Read the model definition and answer for the solid it produces. Units are mm, in the model's axes. A direction names the side the tool comes from. Round coordinates to 2 decimals unless told otherwise and drop trailing zeros. Write each loop counter-clockwise with the first axis right and the second up, starting at its lowest first coordinate (ties: lowest second). Pieces come first, ordered by that corner, then holes. Notation, with made-up numbers: (-17.75, 6.25) - (38.25, 6.25) arc R18 cw to (38.25, 28.25) - close; hole circle Ø1 at (-20.75, -27.75). An arc over 180 degrees is marked (long way). One line per item, written item: value. Start each with the question number.
(1) The mould has two halves that part along Y. Classify faces 1 (the face through (-35.587, -15.804, 3.451)), 2 (the face through (37.801, -21.974, 3.451)), 3 (the face through (1.2, -13.95, 3.45)): +Y half, -Y half, draft (parallel to the pull), parting line (faces both ways), or undercut.
(2) A cutting plane is placed at C-C, the plane x = -30. Determine the outline of the cut face in (y, z), plus the area to 3 significant figures.
(3) Flat-ended cylindrical pins translate along their axes: pin 1 Ø1.5 at (y, z) = (4.5, 5.5) entering from +X; pin 2 Ø1.5 at (y, z) = (1.5, 2) entering from +X; pin 3 Ø3 at (y, z) = (36, 6) entering from -X. Find the tip coordinate at first contact, or state that the pin passes through.
(4) Find the intervals of material crossed by L1, parallel to X at y = 1.5, z = 1.5; L2, parallel to X at y = 24, z = 5.5; L3, parallel to X at y = -15, z = 1, in increasing order.
(5) For faces 4 (the face through (8.566, -17.341, 3.451)), 5 (the face through (-16.806, -14.44, 3.451)), 6 (the face through (12.26, 6.76, 3.45)), determine the directions among +Z, -Z, +X, -X, +Y, -Y from which every point of the face is accessible in a straight line to the end or side of a thin tool.
(6) A cutting plane is placed at A-A, the plane z = 3.75. State how many separate pieces and enclosed holes the cut face has, plus the area to 3 significant figures.
(7) A cutting plane is placed at B-B, the plane x = 32. Determine the outline of the cut face in (y, z).
from build123d import *

# Parameters (mm, degrees)
F1_DEPTH  = 7
F1_FACE_R = 11
F3_DEPTH  = 45.5


with BuildPart() as f1:
    # F0 (on Top) → F1 (new body)
    with BuildSketch(Plane.XY):
        with BuildLine():
            ThreePointArc((-2.885217, -13.699472), (-1.450413, -13.924665), (0, -14))
            ThreePointArc((0, -14), (1.212509, -13.947395), (2.415907, -13.789974))
            Line((2.415907, -13.789974), (14.89071, -20.992305))
            ThreePointArc((14.89071, -20.992305), (37.998969, -21.627676), (25.088992, -2.451445))
            Line((25.088992, -2.451445), (13.306699, 4.351065))
            ThreePointArc((13.306699, 4.351065), (12.242078, 6.792019), (10.734515, 8.987224))
            Line((10.734515, 8.987224), (10.734515, 23.391886))
            ThreePointArc((10.734515, 23.391886), (0, 43.724702), (-10.734515, 23.391886))
            ThreePointArc((-10.734515, 23.391886), (-10.576305, 23.173866), (-10.421482, 22.953427))
            Line((-10.421482, 22.953427), (-10.421482, 9.348407))
            ThreePointArc((-10.421482, 9.348407), (-12.0031, 7.205941), (-13.150422, 4.802751))
            Line((-13.150422, 4.802751), (-25.625225, -2.39958))
            ThreePointArc((-25.625225, -2.39958), (-37.729602, -22.094234), (-14.66751, -20.501982))
            Line((-14.66751, -20.501982), (-2.885217, -13.699472))
        make_face()
        with BuildLine():
            ThreePointArc((0, -11), (-7.778175, 7.778175), (11, 0))
            ThreePointArc((11, 0), (7.778175, -7.778175), (0, -11))
        make_face(mode=Mode.SUBTRACT)
    extrude(amount=F1_DEPTH)

    # F2 (on Top) + F1_face (on face) → F3 (cut)
    with BuildSketch(Plane.XY):
        Polygon((-25.32137, -25.958319), (-16.374294, -19.782603), (-17.249084, -8.94635), (-27.070949, -4.285813), (-36.018025, -10.46153), (-35.143235, -21.297783), align=None)
        Polygon((36.897277, -17.812624), (33.407967, -7.516298), (22.746431, -5.389966), (15.574206, -13.559961), (19.063516, -23.856288), (29.725052, -25.98262), align=None)
        Polygon((5.435753, 40.696717), (-5.435753, 40.696717), (-10.871506, 31.281717), (-5.435753, 21.866717), (5.435753, 21.866717), (10.871506, 31.281717), align=None)
    with BuildSketch(Plane(origin=(8e-06, -1.8e-05, 7), x_dir=(1, 0, 0), z_dir=(0, 0, 1))):
        with BuildLine():
            Line((-14.667518, -20.501964), (-2.885225, -13.699454))
            ThreePointArc((-2.885225, -13.699454), (-0.238987, -13.997942), (2.415899, -13.789957))
            Line((2.415899, -13.789957), (14.890702, -20.992287))
            ThreePointArc((14.890702, -20.992287), (37.998961, -21.627658), (25.088984, -2.451427))
            Line((25.088984, -2.451427), (13.306691, 4.351083))
            ThreePointArc((13.306691, 4.351083), (12.24207, 6.792037), (10.734507, 8.987242))
            Line((10.734507, 8.987242), (10.734507, 23.391904))
            ThreePointArc((10.734507, 23.391904), (-8e-06, 43.72472), (-10.734523, 23.391904))
            ThreePointArc((-10.734523, 23.391904), (-10.576313, 23.173884), (-10.42149, 22.953445))
            Line((-10.42149, 22.953445), (-10.42149, 9.348425))
            ThreePointArc((-10.42149, 9.348425), (-12.003108, 7.205959), (-13.15043, 4.802769))
            Line((-13.15043, 4.802769), (-25.625233, -2.399562))
            ThreePointArc((-25.625233, -2.399562), (-37.72961, -22.094217), (-14.667518, -20.501964))
        make_face()
        with Locations((-8e-06, 1.8e-05)):
            Circle(F1_FACE_R, mode=Mode.SUBTRACT)
    extrude(amount=F3_DEPTH, mode=Mode.SUBTRACT)


solid = f1.part
Here are the results:
1. face 1: undercut
1. face 2: parting line
1. face 3: -Y half
2. outline: (-27.91, 0) - (-23.74, 0) - (-23.74, 7) - (-27.91, 7) - close; (-6.31, 0) - (-2.81, 0) - (-2.81, 7) - (-6.31, 7) - close
2. area: 53.7 mm²
3. pin 1: x = 14.35
3. pin 2: x = 19.54
3. pin 3: x = -12.44
4. L1: -18.87 to -10.9, 10.9 to 18.24
4. L2: -11.13 to -6.67, 6.67 to 11.13
4. L3: -39.6 to -35.65, -16.76 to -5.14, 4.51 to 16.06, 35.94 to 39.6
5. face 4: +Z, -Z, -Y
5. face 5: +Z, -Z
5. face 6: +Z, -Z, +X
6. separate pieces: 1
6. enclosed holes: 4
6. area: 1,340 mm²
7. outline: (-27.19, 0) - (-23.39, 0) - (-23.39, 7) - (-27.19, 7) - close; (-7.24, 0) - (-3.53, 0) - (-3.53, 7) - (-7.24, 7) - close
